Check sheet for the modelled part. Datum: model origin and axes. Units: mm. Face numbers are marked on the shaded views. A direction names the side the tool comes from. Round coordinates to 2 decimals unless told otherwise and drop trailing zeros. Order: outer loops, then holes, each group sorted by start corner. A loop starts at its lowest first (then second) coordinate and runs counter-clockwise, first axis right, second up. Notation, with made-up numbers: (55.5, 58.5) -> (91.5, 58.5) arc R35 ccw to (91.5, 94.5) -> close; hole circle Ø3 at (18.5, -3). An arc over 180 degrees is marked (long way). Answer in a Markdown table with one row per item.
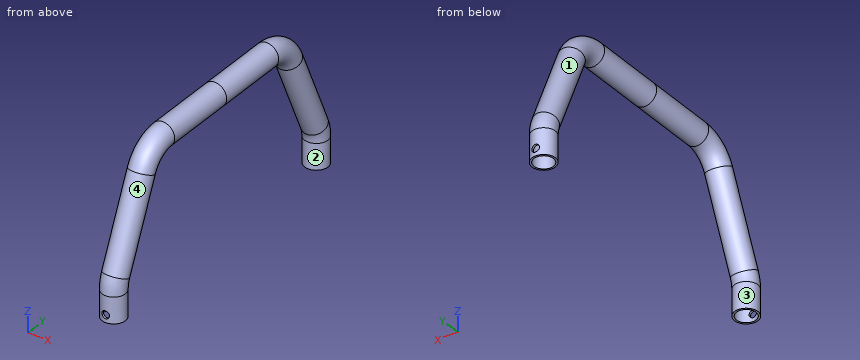
```python
from build123d import *

# Parameters (mm, degrees)
F1_R     = 12.5
F1_R_2   = 10.5
F4_R     = 4
F5_DEPTH = 12.5010001


with BuildPart() as f2:
    # F2: sweep along a path in F0
    with BuildLine(Plane.YZ) as f2_path:
        Line((0, 150), (-77.0523680748, 150))
        ThreePointArc((-77.0523680748, 150), (-96.2429974746, 144.269775251), (-109.1498200437, 128.9554138995))
        Line((-109.1498200437, 128.9554138995), (-147.0974519689, 41.6758604716))
        ThreePointArc((-147.0974519689, 41.6758604716), (-149.2666807476, 34.8474789521), (-150, 27.7204465721))
        Line((-150, 27.7204465721), (-150, 0))
    # F1 (on Top) → F2 (sweep)
    with BuildSketch(Plane.XY):
        with Locations((0, -150)):
            Circle(F1_R)
        with Locations((0, -150)):
            Circle(F1_R_2, mode=Mode.SUBTRACT)
    sweep(path=f2_path.line)

    # F4 (on plane+point) → F5 (cut, through all)
    with BuildSketch(Plane.XZ.offset(150)):
        with Locations((0, 8)):
            Circle(F4_R)
    extrude(amount=F5_DEPTH, mode=Mode.SUBTRACT)

    # F6: F2 across plane


with BuildPart() as f2_1:
    add(f2.part)
    add(f2.part.mirror(Plane.XZ))


solid = f2_1.part
```
(1) Depth check by flat-ended pin: pin 1 Ø1 at (x, y) = (-5, 3.5) entering from -Z; pin 2 Ø2 at (x, y) = (4.5, -77.5) entering from -Z; pin 3 Ø12.5 at (x, z) = (0, 150) entering from +Y. Enter the tip coordinate at first touch or a pass-through.
Solutions:
| item | result |
|---|---|
| pin 1 | z = 138.34 |
| pin 2 | z = 137.99 |
| pin 3 | y = 114.86 |
(2) Scan lines: probe 1 along Y at (x, z) = (0, 10.5); probe 2 along Y at (x, z) = (0.25, 131.5); probe 3 along X at (y, z) = (150, 11). Record each from-to range of solid material in increasing order. Write a range as from..to.
Solutions:
| item | result |
|---|---|
| probe 1 | -139.5..-137.5, 137.5..139.5 |
| probe 2 | -121.67..-119.49, -95.17..-92.35, 92.35..95.17, 119.49..121.67 |
| probe 3 | -12.5..-10.5, 10.5..12.5 |
(3) Section check A-A on y = -71.5. Record the boundary of the cut face in (x, z).
Solutions:
| item | result |
|---|---|
| outline | circle Ø25 at (0, 150); hole circle Ø21 at (0, 150) |
(4) Tool access check on the marked faces 3 and 4. Record the directions out of +Z, -Z, +X, -X, +Y, -Y that give a thin tool (end or side, any length) a straight path to the whole face; none if there is none.
Solutions:
| item | result |
|---|---|
| face 3 | -Z |
| face 4 | none |
(5) Draft check along Y on the marked faces 1 and 2. Enter one of: pulls with the +Y half, pulls with the -Y half, needs draft (parallel to the pull), parting line crosses it, or undercut.
Solutions:
| item | result |
|---|---|
| face 1 | undercut |
| face 2 | undercut |
(6) Section check C-C on x = 0. Give the number of separate pieces and of enclosed holes in the cut face, plus the area to 3 significant figures.
Solutions:
| item | result |
|---|---|
| separate pieces | 4 |
| enclosed holes | 0 |
| area | 2,010 mm^2 |
(7) Section check B-B on z = 24.5. Record the boundary of the cut face in (x, y).
Solutions:
| item | result |
|---|---|
| outline | circle Ø25 at (0, -150); circle Ø25 at (0, 150); hole circle Ø21 at (0, -150); hole circle Ø21 at (0, 150) |
